from build123d import *

# Parameters (mm, degrees)
BOSS_EXTRUDE1_DEPTH = 7.32


with BuildPart() as part:
    # Sketch1 → Boss-Extrude1 (new body)
    with BuildSketch(Plane.XY):
        Polygon((0, 10.779129526), (-9.335, 5.389564763), (-9.335, -5.389564763), (0, -10.779129526), (9.335, -5.389564763), (9.335, 5.389564763), align=None)
    extrude(amount=BOSS_EXTRUDE1_DEPTH)

    # Sketch2 → Revolve1 (revolve)
    with BuildSketch(Plane(origin=(0, 0, 0), x_dir=(0, 0, -1), z_dir=(1, 0, 0))):
        with BuildLine():
            Line((0, 0), (0, 6.6))
            ThreePointArc((0, 6.6), (0.175735931, 6.175735931), (0.6, 6))
            Line((0.6, 6), (109.1, 6))
            Line((109.1, 6), (110, 5.1))
            Line((110, 5.1), (110, 0))
            Line((110, 0), (0, 0))
        make_face()
    revolve(axis=Axis((0, 0, 0), (0, 0, -1)))

    # Sketch3 → Cut-Revolve1 (revolve, cut)
    with BuildSketch(Plane(origin=(0, 0, 0), x_dir=(0, 0, -1), z_dir=(1, 0, 0))):
        Polygon((-7.32, 10.779129526), (-6.48623143, 10.779129526), (-7.32, 9.335), align=None)
        Polygon((-0.15, 10.779129526), (-0.15, 8.78660254), (0, 8.7), (0, 10.779129526), align=None)
    revolve(axis=Axis((0, 0, 12.204941078), (0, 0, -1)), mode=Mode.SUBTRACT)


solid = part.part
Verification items for the finished model (mm, model axes). A direction names the side the tool comes from. Coordinates: 2 decimals unless noted, no trailing zeros. Order: outer loops, then holes, each group sorted by start corner. A loop starts at its lowest first (then second) coordinate and runs counter-clockwise, first axis right, second up. Notation, with made-up numbers: M 56,-30 L 77,-30 A22 cw 77,-3 Z; hole C -5,-22 d10. An arc over 180 degrees is marked long. Return JSON: item names as keys, results as strings.
1) Access from +Z, -Z, +X, -X, +Y, -Y to the whole of each face (thin tool, end or side, straight path). Record for faces 1 (the flat face through (0, 0, -110)), 2 (the flat face through (-6.5, 2, 0)).
Answer list:
{"face 1": "-Z, +X, -X, +Y, -Y", "face 2": "-Z"}
2) Cross-section at A-A, the plane z = -99. Record the boundary of the cut face in (x, y).
Answer list:
{"outline": "C 0,0 d12"}
3) Gauge pin test, flat ends, axial feed: pin 1 (8 mm diameter, centred on y = -1, z = -84.5, fed in from -X); pin 2 (12 mm diameter, centred on y = -3, z = -11.5, fed in from +X); pin 3 (1.5 mm diameter, centred on y = -2, z = -30.5, fed in from +X); pin 4 (3 mm diameter, centred on x = 7, y = -8, fed in from +Z). Record the tip position at first contact, or that the pin passes through.
Answer list:
{"pin 1": "x = -6", "pin 2": "x = 6", "pin 3": "x = 5.87", "pin 4": "z = 7.32"}
4) Thickness scan on L1, parallel to Z at x = -6.25, y = 5; L2, parallel to X at y = 0.5, z = -13; L3, parallel to Y at x = -5, z = -32.5. Record the ranges inside material, lowest first. Write a range as [from, to].
Answer list:
{"L1": "[0, 7.32]", "L2": "[-5.98, 5.98]", "L3": "[-3.32, 3.32]"}
